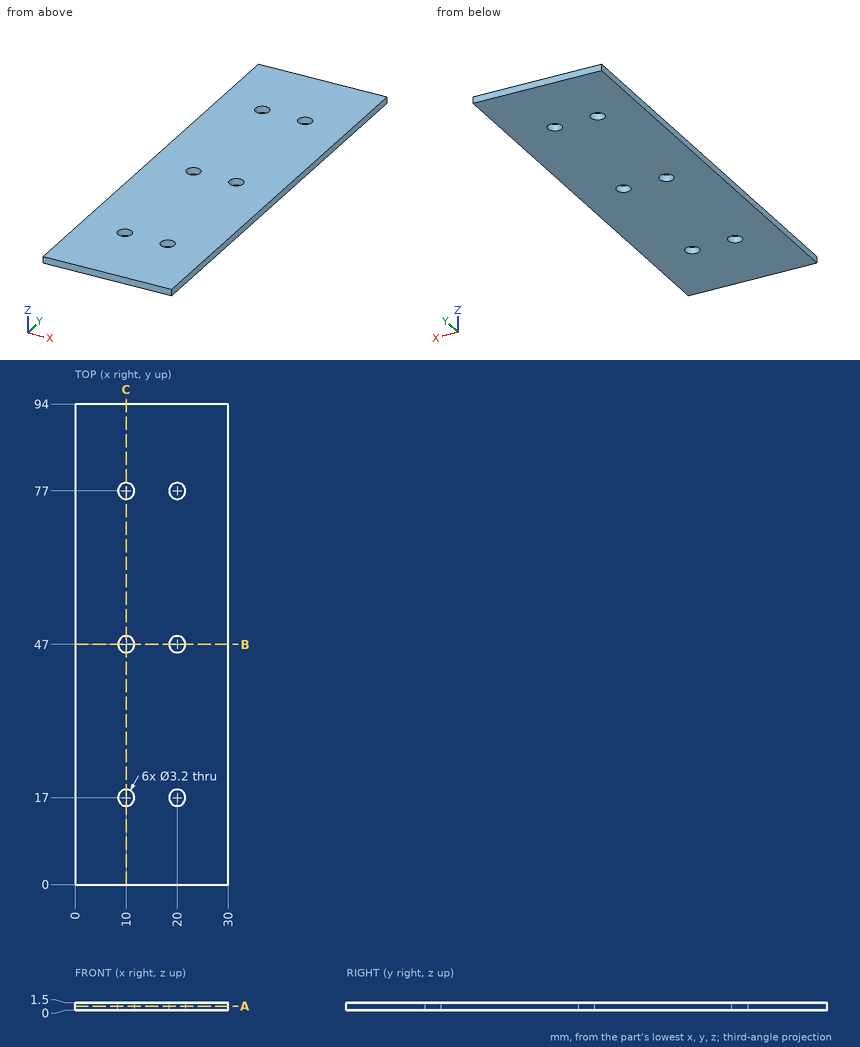
Geometry: see drawing. Coordinates: mm, zero at the bounding-box minimum. Give positions to 0.01 mm unless a question says otherwise; leave off trailing zeros. Loops run counter-clockwise (first coordinate to the right, second up) from the corner with the lowest first, then second, coordinate; pieces in that order, holes last. Notation, with made-up numbers: (55, 48) - (95, 48) arc R33 ccw to (95, 85) - close; hole circle Ø5 at (14, 87.25). An arc over 180 degrees is marked (long way). Use CSV: the item, a comma, the result in double quotes.
1) Pin query (flat end, axial travel): P1, Ø2.5, axis at x = 10, y = 77, coming from the +Z side. Return the tip coordinate at first contact, or that it passes through.
Worked out:
P1,"passes through"
2) Cut plane B-B (y = 47). Output: boundary loops of the cut face in (x, z).
Worked out:
outline,"(0, 0) - (8.4, 0) - (8.4, 1.5) - (0, 1.5) - close; (11.6, 0) - (18.4, 0) - (18.4, 1.5) - (11.6, 1.5) - close; (21.6, 0) - (30, 0) - (30, 1.5) - (21.6, 1.5) - close"
3) Cut plane C-C (x = 10). Output: boundary loops of the cut face in (y, z), and give its area (3 significant figures).
Worked out:
outline,"(0, 0) - (15.4, 0) - (15.4, 1.5) - (0, 1.5) - close; (18.6, 0) - (45.4, 0) - (45.4, 1.5) - (18.6, 1.5) - close; (48.6, 0) - (75.4, 0) - (75.4, 1.5) - (48.6, 1.5) - close; (78.6, 0) - (94, 0) - (94, 1.5) - (78.6, 1.5) - close"
area,"127 mm^2"
4) Cut plane A-A (z = 0.8). Output: boundary loops of the cut face in (x, y).
Worked out:
outline,"(0, 0) - (30, 0) - (30, 94) - (0, 94) - close; hole circle Ø3.2 at (10, 17); hole circle Ø3.2 at (10, 47); hole circle Ø3.2 at (10, 77); hole circle Ø3.2 at (20, 17); hole circle Ø3.2 at (20, 47); hole circle Ø3.2 at (20, 77)"
5) Line query: line 1 (Y direction, x = 10, z = 0.4); line 2 (X direction, y = 78, z = 0.75); line 3 (X direction, y = 47.5, z = 0.7). Output: solid intervals per line, ascending.
Worked out:
line 1,"y = 0 to 15.4, 18.6 to 45.4, 48.6 to 75.4, 78.6 to 94"
line 2,"x = 0 to 8.75, 11.25 to 18.75, 21.25 to 30"
line 3,"x = 0 to 8.48, 11.52 to 18.48, 21.52 to 30"
